The figure shows three views and two pictorial views of one solid part (mm, origin at its lowest corner). Answer the questions. A direction names the side the tool comes from. Give positions to 0.01 mm unless a question says otherwise; leave off trailing zeros. Loops run counter-clockwise (first coordinate to the right, second up) from the corner with the lowest first, then second, coordinate; pieces in that order, holes last. Notation, with made-up numbers: (-18.5, 76.25) - (2.5, 76.25) arc R8 cw to (2.5, 89.25) - close; hole circle Ø11 at (15.5, 58). An arc over 180 degrees is marked (long way). Use a Markdown table: item, result. Add a question column.
Item 1: Consider probe 1 along Z at (x, y) = (6.75, 10.75); probe 2 along Y at (x, z) = (7.75, 23); probe 3 along Y at (x, z) = (14.25, 29) (1 decimal). Determine where each line is inside the solid, lowest interval first. Write a range as [from, to].
Item 2: Which of the six approach directions +Z, -Z, +X, -X, +Y, -Y give full straight-line access (tool end or side, diameter ignored) to the marked faces 1 and 2?
Item 3: A cutting plane is placed at D-D (y = 11.5). Determine the outline of the cut face in (x, z) (1 decimal).
Item 4: A cutting plane is placed at A-A (y = 8.75). Determine the outline of the cut face in (x, z), plus the area to 3 significant figures.
Item 5: A cutting plane is placed at C-C (z = 7). Determine the outline of the cut face in (x, y) (1 decimal).
Item 6: A cutting plane is placed at B-B (x = 13.5). Determine the outline of the cut face in (y, z).
Item 7: Each of these flat-tipped pins is pushed along its axis until it touches: P1, Ø1, axis at y = 2.5, z = 8, coming from the +X side; P2, Ø4, axis at x = 12.5, y = 1.5, coming from the -Z side; P3, Ø5, axis at x = 4.5, z = 3.5, coming from the -Y side. Where does it stop, or does it pass through?
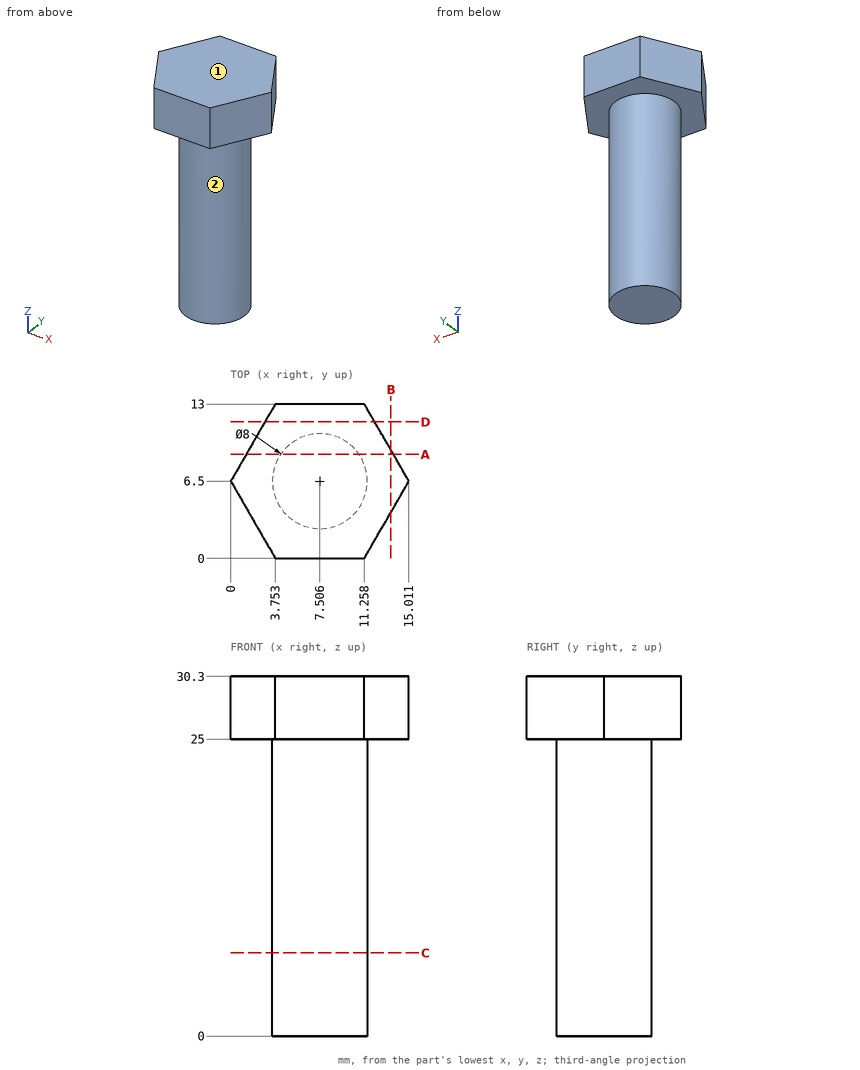
Geometry says:
| question | item | result |
|---|---|---|
| 1 | probe 1 | [25, 30.3] |
| 1 | probe 2 | [2.51, 10.49] |
| 1 | probe 3 | [5.2, 7.8] |
| 2 | face 1 | +Z, +X, -X, +Y, -Y |
| 2 | face 2 | -Z |
| 3 | outline | (2.9, 25) - (12.1, 25) - (12.1, 30.3) - (2.9, 30.3) - close |
| 4 | outline | (1.3, 25) - (4.2, 25) - (4.2, 0) - (10.81, 0) - (10.81, 25) - (13.71, 25) - (13.71, 30.3) - (1.3, 30.3) - close |
| 4 | area | 231 mm² |
| 5 | outline | circle Ø8 at (7.5, 6.5) |
| 6 | outline | (3.88, 25) - (9.12, 25) - (9.12, 30.3) - (3.88, 30.3) - close |
| 7 | P1 | x = 9.44 |
| 7 | P2 | z = 25 |
| 7 | P3 | y = 2.53 |
